Verification items for the finished model (mm, model axes). Face numbers are marked on the shaded views. Give positions to 0.01 mm unless a question says otherwise; leave off trailing zeros. Order: outer loops, then holes, each group sorted by start corner. A loop starts at its lowest first (then second) coordinate and runs counter-clockwise, first axis right, second up. Notation, with made-up numbers: M -36,40.5 L 21,40.5 A15 ccw 21,63.5 Z; hole C -35.5,40 d8. An arc over 180 degrees is marked long. Answer as a JSON object with one key per item and string values.
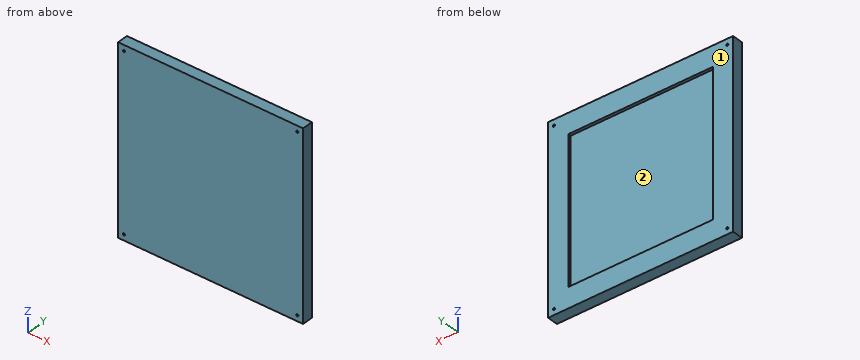
```python
from build123d import *

# Parameters (mm, degrees)
F0_W          = 812.8
F0_H          = 812.8
F0_W_2        = 635
F0_H_2        = 635
F1_DEPTH      = 38.1
F3_W          = 812.8
F3_H          = 812.8
F4_DEPTH      = 9.525
F4_DEPTH_BACK = 25.4
F5_R          = 4.7625
F6_DEPTH      = 254


with BuildPart() as f1:
    # F0 (on Front) → F1 (new body)
    with BuildSketch(Plane.XZ):
        Rectangle(F0_W, F0_H)
        Rectangle(F0_W_2, F0_H_2, mode=Mode.SUBTRACT)
    extrude(amount=F1_DEPTH)

    # F3 (on face) → F4 (join, two sides)
    with BuildSketch(Plane.XZ.offset(38.1)) as f4_sk:
        Rectangle(F3_W, F3_H)
    extrude(amount=F4_DEPTH)
    extrude(f4_sk.sketch, amount=-F4_DEPTH_BACK)

    # F5 (on face) → F6 (cut)
    with BuildSketch(Plane(origin=(0, 0, 0), x_dir=(-1, 0, 0), z_dir=(0, 1, 0))):
        with Locations((-381, -381)):
            Circle(F5_R)
        with Locations((381, -381)):
            Circle(F5_R)
        with Locations((381, 381)):
            Circle(F5_R)
        with Locations((-381, 381)):
            Circle(F5_R)
    extrude(amount=-F6_DEPTH, mode=Mode.SUBTRACT)


solid = f1.part
```
Q1. Gauge pin test, flat end, axial feed: pin 1 Ø4 at (x, z) = (-88.5, -1) entering from +Y. Record the tip position at first contact, or that the pin passes through.
Resolved:
{"pin 1": "stops at y = -12.7"}
Q2. Release check for a two-part mould opening along X. For the marked faces 1 and 2 record: +X half, -X half, draft (parallel to the pull), parting line (faces both ways), or undercut.
Resolved:
{"face 1": "draft", "face 2": "undercut"}
Q3. Material ranges on L1, parallel to Z at x = -381, y = -28; L2, parallel to X at y = -7.5, z = 6.5, recorded low to high.
Resolved:
{"L1": "z = -406.4 to -385.76, -376.24 to 376.24, 385.76 to 406.4", "L2": "x = -406.4 to -317.5, 317.5 to 406.4"}
Q4. Section check A-A on x = 49. Record the cut outline in (y, z) (3 decimals).
Resolved:
{"outline": "M -47.625,-406.4 L 0,-406.4 L 0,-317.5 L -12.7,-317.5 L -12.7,317.5 L 0,317.5 L 0,406.4 L -47.625,406.4 Z"}
Q5. Section check B-B on z = 9. Record the cut outline in (x, y) (3 decimals).
Resolved:
{"outline": "M -406.4,-47.625 L 406.4,-47.625 L 406.4,0 L 317.5,0 L 317.5,-12.7 L -317.5,-12.7 L -317.5,0 L -406.4,0 Z"}
